Part model, mm, in its own coordinate system. A direction names the side the tool comes from. Round coordinates to 2 decimals unless told otherwise and drop trailing zeros. Loops run counter-clockwise (first coordinate to the right, second up) from the corner with the lowest first, then second, coordinate; pieces in that order, holes last. Notation, with made-up numbers: (39.25, 36.25) -> (98.25, 36.25) arc R8 cw to (98.25, 47.25) -> close; hole circle Ø7 at (52.25, -13.75). An arc over 180 degrees is marked (long way). Answer as CSV lines item,"result".
from build123d import *

# Parameters (mm, degrees)
F0_R          = 3.937
F1_DEPTH      = 101.6
F1_DEPTH_BACK = 2.54
F0_R_2        = 9.144
F2_DEPTH      = 4.7625


# Not quite as in the source:
# - a fillet or chamfer that OpenCascade refuses, or shapes differently, is made with other operations: its cross-section is extruded or revolved along the edge and cut away or added


with BuildPart() as f1:
    # F0 (on Top) → F1 (new body, two sides)
    with BuildSketch(Plane.XY) as f1_sk:
        Circle(F0_R)
    extrude(amount=F1_DEPTH)
    extrude(f1_sk.sketch, amount=-F1_DEPTH_BACK)

    # F0 (on Top) → F2 (join)
    with BuildSketch(Plane.XY):
        Circle(F0_R_2)
        Circle(F0_R, mode=Mode.SUBTRACT)
        Circle(F0_R)
    extrude(amount=-F2_DEPTH)

    # F3: fillet of radius 5.08 on 1 edges, made by hand

    # F3_s1 → F3_t2 (revolve, cut)
    with BuildSketch(Plane.XZ):
        with BuildLine():
            ThreePointArc((9.144, 0), (7.5519698235, -3.3851544532), (4.0739315833, -4.7625))
            Line((4.0739315833, -4.7625), (9.144, -4.7625))
            Line((9.144, -4.7625), (9.144, 0))
        make_face()
    revolve(axis=Axis((0, 0, -4.7625), (0, 0, 1)), mode=Mode.SUBTRACT)


solid = f1.part
Q1. Saw through at A-A, the plane z = 62. Write the cut outline in (x, y).
Geometry results:
outline,"circle Ø7.87 at (0, 0)"
Q2. Drill centre lines: line 1 along Z through (x, y) = (-7.5, -0.5); line 2 along Z through (x, y) = (-0.25, -5.25); line 3 along Y through (x, z) = (2.25, 30.5). Where is each one in solid material? Low to high.
Geometry results:
line 1,"-3.42 to 0"
line 2,"-4.62 to 0"
line 3,"-3.23 to 3.23"
Q3. Which spindle directions (+Z, -Z, +X, -X, +Y, -Y) get a long thin tool onto all of the face, cutting with end or side? Do faces 1 (the face through (0, 0, -4.762)), 2 (the face through (4, -2, 0)). Say none if no direction does.
Geometry results:
face 1,"-Z, +X, -X, +Y, -Y"
face 2,"+Z"
Q4. Drop flat-ended pins along their axis: P1, Ø6, axis at x = -4.5, y = -2, coming from the -Z side; P2, Ø6, axis at x = 3.5, z = 48, coming from the -Y side; P3, Ø8, axis at x = 5, z = 20.5, coming from the +Y side; P4, Ø5, axis at x = -3.5, y = -6, coming from the -Z side. Give the stop position or say it passes through.
Geometry results:
P1,"z = -4.76"
P2,"y = -3.91"
P3,"y = 3.81"
P4,"z = -4.75"
